```python
from build123d import *

# Parameters (mm, degrees)
CROQUIS1_W              = 50
CROQUIS1_H              = 50
CROQUIS1_W_2            = 47.6
CROQUIS1_H_2            = 47.6
SALIENTE_EXTRUIR1_DEPTH = 237
CROQUIS2_R              = 2.5
CROQUIS2_R_2            = 3.5
CORTAR_EXTRUIR1_DEPTH   = 244.503593403
CHAFL_N1_SIZE           = 1
CROQUIS3_R              = 4
CORTAR_EXTRUIR2_DEPTH   = 244.503593403
CROQUIS4_R              = 9
CORTAR_EXTRUIR3_DEPTH   = 244.503593403
CROQUIS5_R              = 2.5
CORTAR_EXTRUIR4_DEPTH   = 2


with BuildPart() as part:
    # Croquis1 → Saliente-Extruir1 (new body)
    with BuildSketch(Plane.XY):
        Rectangle(CROQUIS1_W, CROQUIS1_H)
        Rectangle(CROQUIS1_W_2, CROQUIS1_H_2, mode=Mode.SUBTRACT)
    extrude(amount=SALIENTE_EXTRUIR1_DEPTH)

    # Croquis2 → Cortar-Extruir1 (cut, through all)
    with BuildSketch(Plane(origin=(25, 0, 0), x_dir=(0, 0, -1), z_dir=(1, 0, 0))):
        with Locations(Location((-10, 19, 0), (0, 0, 90))):
            Circle(CROQUIS2_R)
        with Locations(Location((-25, 19, 0), (0, 0, 90))):
            Circle(CROQUIS2_R)
        with Locations(Location((-25, -19, 0), (0, 0, 90))):
            Circle(CROQUIS2_R)
        with Locations(Location((-10, -19, 0), (0, 0, 90))):
            Circle(CROQUIS2_R)
        with Locations(Location((-227, 19, 0), (0, 0, 90))):
            Circle(CROQUIS2_R)
        with Locations(Location((-212, 19, 0), (0, 0, 90))):
            Circle(CROQUIS2_R)
        with Locations(Location((-212, -19, 0), (0, 0, 90))):
            Circle(CROQUIS2_R)
        with Locations(Location((-227, -19, 0), (0, 0, 90))):
            Circle(CROQUIS2_R)
        with Locations(Location((-220, 0, 0), (0, 0, 90))):
            Circle(CROQUIS2_R_2)
    extrude(amount=-CORTAR_EXTRUIR1_DEPTH, mode=Mode.SUBTRACT)

    # Chaflán1
    chafl_n1_edges = [part.edges().sort_by_distance(p)[0] for p in [
        (0, -25, 0),
        (-25, 0, 0),
        (0, 25, 0),
        (25, 0, 0),
    ]]
    chamfer(chafl_n1_edges, length=CHAFL_N1_SIZE)

    # Croquis3 → Cortar-Extruir2 (cut, through all)
    with BuildSketch(Plane(origin=(0, 25, 0), x_dir=(1, 0, 0), z_dir=(0, 1, 0))):
        with Locations(Location((0, -220, 0), (0, 0, 270))):
            Circle(CROQUIS3_R)
    extrude(amount=-CORTAR_EXTRUIR2_DEPTH, mode=Mode.SUBTRACT)

    # Croquis4 → Cortar-Extruir3 (cut, through all)
    with BuildSketch(Plane(origin=(0, 25, 0), x_dir=(1, 0, 0), z_dir=(0, 1, 0))):
        with Locations(Location((0, -167, 0), (0, 0, 270))):
            Circle(CROQUIS4_R)
    extrude(amount=-CORTAR_EXTRUIR3_DEPTH, mode=Mode.SUBTRACT)

    # Croquis5 → Cortar-Extruir4 (cut)
    with BuildSketch(Plane(origin=(0, 25, 0), x_dir=(1, 0, 0), z_dir=(0, 1, 0))):
        with Locations(Location((-15, -136, 0), (0, 0, 270))):
            Circle(CROQUIS5_R)
        with Locations(Location((15, -136, 0), (0, 0, 270))):
            Circle(CROQUIS5_R)
        with Locations(Location((-15, -198, 0), (0, 0, 270))):
            Circle(CROQUIS5_R)
        with Locations(Location((15, -198, 0), (0, 0, 270))):
            Circle(CROQUIS5_R)
    extrude(amount=-CORTAR_EXTRUIR4_DEPTH, mode=Mode.SUBTRACT)


solid = part.part
```
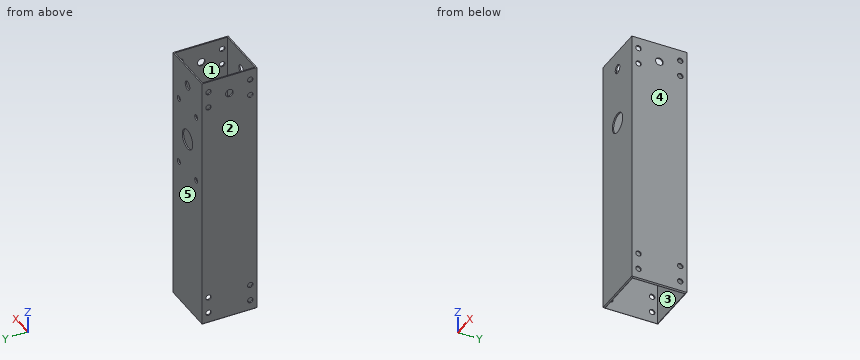
Verification items for the finished model (mm, model axes). Face numbers are marked on the shaded views. A direction names the side the tool comes from. Round coordinates to 2 decimals unless told otherwise and drop trailing zeros. Write each loop counter-clockwise with the first axis right and the second up, starting at its lowest first coordinate (ties: lowest second). Pieces come first, ordered by that corner, then holes. Notation, with made-up numbers: (44, 63.25) -> (96, 63.25) arc R22 cw to (96, 94.25) -> close; hole circle Ø10 at (42.25, 88.25). An arc over 180 degrees is marked (long way). Write each question's results on one line, items separated by ' | '. Start each with the question number.
1. Material ranges on probe 1 along X at (y, z) = (24.3, 136); probe 2 along Z at (x, y) = (24, 19); probe 3 along X at (y, z) = (1.5, 123), recorded low to high. Write a range as from..to.
2. Cross-section at C-C (x = 0). Enter the section's corners in (y, z).
3. Cross-section at A-A (z = 227). Enter the section's corners in (x, y), then the cut area to 3 significant figures.
4. Depth check by flat-ended pin: P1, Ø4, axis at y = 19, z = 212, coming from the +X side. Enter the tip coordinate at first touch or a pass-through.
5. Draft check along Y on the marked faces 3, 4 and 5. Enter one of: +Y half, -Y half, draft (parallel to the pull), parting line (faces both ways), or undercut.
6. Set-up check for the marked faces 1 and 2: record each of +Z, -Z, +X, -X, +Y, -Y from which the full face is reachable in a straight line by a thin tool's end or side.
7. Cross-section at D-D (y = -9). Enter the section's corners in (x, z), then the cut area to 3 significant figures.
8. Cross-section at B-B (z = 122.5). Enter the section's corners in (x, y).
Solutions:
1) probe 1: x = -25..-17.5, -12.5..12.5, 17.5..25 | probe 2: z = 0..7.5, 12.5..22.5, 27.5..209.5, 214.5..224.5, 229.5..237 | probe 3: x = -25..-23.8, 23.8..25
2) outline: (-25, 1) -> (-24, 0) -> (-23.8, 0) -> (-23.8, 158) -> (-25, 158) -> close; (-25, 176) -> (-23.8, 176) -> (-23.8, 216) -> (-25, 216) -> close; (-25, 224) -> (-23.8, 224) -> (-23.8, 237) -> (-25, 237) -> close; (23.8, 0) -> (24, 0) -> (25, 1) -> (25, 158) -> (23.8, 158) -> close; (23.8, 176) -> (25, 176) -> (25, 216) -> (23.8, 216) -> close; (23.8, 224) -> (25, 224) -> (25, 237) -> (23.8, 237) -> close
3) outline: (-25, -25) -> (25, -25) -> (25, -21.5) -> (23.8, -21.5) -> (23.8, -23.8) -> (-23.8, -23.8) -> (-23.8, -21.5) -> (-25, -21.5) -> close; (-25, -16.5) -> (-23.8, -16.5) -> (-23.8, 16.5) -> (-25, 16.5) -> close; (-25, 21.5) -> (-23.8, 21.5) -> (-23.8, 23.8) -> (23.8, 23.8) -> (23.8, 21.5) -> (25, 21.5) -> (25, 25) -> (-25, 25) -> close; (23.8, -16.5) -> (25, -16.5) -> (25, 16.5) -> (23.8, 16.5) -> close | area: 210 mm2
4) P1: passes through
5) face 3: undercut | face 4: draft | face 5: +Y half
6) face 1: +Z, -Z | face 2: +Z, -Z, -X, +Y, -Y
7) outline: (-25, 1) -> (-24, 0) -> (-23.8, 0) -> (-23.8, 237) -> (-25, 237) -> close; (23.8, 0) -> (24, 0) -> (25, 1) -> (25, 237) -> (23.8, 237) -> close | area: 568 mm2
8) outline: (-25, -25) -> (25, -25) -> (25, 25) -> (-25, 25) -> close; hole (-23.8, -23.8) -> (23.8, -23.8) -> (23.8, 23.8) -> (-23.8, 23.8) -> close
